Work out the finished part from the listing and answer in its coordinate system (mm). A direction names the side the tool comes from. Give positions to 0.01 mm unless a question says otherwise; leave off trailing zeros. Order: outer loops, then holes, each group sorted by start corner. A loop starts at its lowest first (then second) coordinate and runs counter-clockwise, first axis right, second up. Notation, with made-up numbers: M 80,54 L 89,54 A22 ccw 89,79 Z; hole C 30,41.5 d8. An arc over 180 degrees is marked long. One line per item, written item: value.
from build123d import *

# Parameters (mm, degrees)
EXTRUDE1_DEPTH = 9.525
SHELL1_T       = -3.175
SKETCH4_R      = 3.2729084122023364
EXTRUDE2_DEPTH = 3.175
FILLET1_R      = 6.35
FILLET2_R      = 1.016
EXTRUDE3_REACH = 99.642
SKETCH5_R      = 3.633554116992031
SKETCH5_R_2    = 2.5400000000000023
SKETCH6_R      = 2.7088319516261428
SKETCH6_R_2    = 1.739899999999999
EXTRUDE4_DEPTH = 98.64160513278141
FILLET3_R      = 0.508


with BuildPart() as part:
    # Sketch1 → Extrude1 (new body)
    with BuildSketch(Plane(origin=(0, 0, 0), x_dir=(1, 0, 0), z_dir=(0, 1, 0))):
        with BuildLine():
            Line((13.334999999999999, 0), (63.5, 0))
            Line((63.5, 0), (63.5, 38.988999999999926))
            ThreePointArc((63.5, 38.988999999999926), (60.71019209080187, 45.724192090801864), (53.97499999999993, 48.513999999999996))
            Line((53.97499999999993, 48.513999999999996), (0, 48.513999999999996))
            Line((0, 48.513999999999996), (0, 13.334999999999999))
            ThreePointArc((0, 13.334999999999999), (9.429268927122612, 9.42926892712261), (13.334999999999999, 0))
        make_face()
        with BuildLine():
            Line((25.717261934170715, 14.596576467420496), (42.82641557504918, 26.576534819151746))
            ThreePointArc((42.82641557504918, 26.576534819151746), (48.13271108628772, 25.640891752908175), (47.19706802004417, 20.334596241669633))
            Line((47.19706802004417, 20.334596241669633), (30.087914379165696, 8.354637889938386))
            ThreePointArc((30.087914379165696, 8.354637889938386), (24.78161886792715, 9.29028095618195), (25.717261934170715, 14.596576467420496))
        make_face(mode=Mode.SUBTRACT)
    extrude(amount=EXTRUDE1_DEPTH)

    # Shell1
    shell1_openings = [part.faces().sort_by_distance(p)[0] for p in [
        (38.4175, 4.7625, 0),
        (9.429268927, 4.7625, -9.429268927),
        (0, 4.7625, -30.9245),
        (32.524178478, 9.525, -25.566315858),
        (24.781618868, 4.7625, -9.290280956),
        (38.6424912, 4.7625, -14.344617066),
        (48.132711086, 4.7625, -25.640891753),
        (34.271838755, 4.7625, -20.586555643),
    ]]
    offset(amount=SHELL1_T, openings=shell1_openings, kind=Kind.INTERSECTION)

    # Sketch4 → Extrude2 (add)
    with BuildSketch(Plane(origin=(0, 0, 0), x_dir=(1, 0, 0), z_dir=(0, 1, 0))):
        with BuildLine():
            Line((41.325799999999994, 48.513999999999996), (66.82999351166346, 57.21904298473958))
            ThreePointArc((66.82999351166346, 57.21904298473958), (76.90463826764335, 54.01609142946003), (76.79370933191484, 43.445137811366784))
            Line((76.79370933191484, 43.445137811366784), (63.5, 25.8572))
            Line((63.5, 25.8572), (63.5, 38.988999999999926))
            ThreePointArc((63.5, 38.988999999999926), (60.71019209080187, 45.724192090801864), (53.97499999999993, 48.513999999999996))
            Line((53.97499999999993, 48.513999999999996), (41.325799999999994, 48.513999999999996))
        make_face()
        with Locations(Location((69.70164744855023, 48.8056189691106, 0), (0, 0, 270))):
            Circle(SKETCH4_R, mode=Mode.SUBTRACT)
    extrude(amount=EXTRUDE2_DEPTH)

    # Fillet1
    fillet1_edges = [part.edges().sort_by_distance(p)[0] for p in [
        (41.325799999999994, 1.5875, -48.513999999999996),
        (63.5, 1.5875, -25.8572),
    ]]
    fillet(fillet1_edges, radius=FILLET1_R)

    # Fillet2
    fillet2_edges = [part.edges().sort_by_distance(p)[0] for p in [
        (47.12348109415911, 3.175, -48.513999999999996),
        (26.987500000000004, 3.175, -45.339),
        (58.46512806053458, 3.175, -43.47912806053458),
        (60.325, 3.175, -19.494500000000002),
        (60.71019209080187, 3.175, -45.724192090801864),
        (63.5, 3.175, -31.358185610352162),
    ]]
    fillet(fillet2_edges, radius=FILLET2_R)

    # Sketch5 → Extrude3 (add, up to next)
    with BuildSketch(Plane(origin=(0, 4.191000000000001, 0), x_dir=(-1, 0, 0), z_dir=(0, 1, 0)), mode=Mode.PRIVATE) as extrude3_sk1:
        with Locations(Location((-53.334326567522815, -29.283102123737322, 0), (0, 0, 90))):
            Circle(SKETCH5_R)
    extrude3_tool1 = extrude(extrude3_sk1.sketch, amount=-EXTRUDE3_REACH, mode=Mode.PRIVATE) - part.part
    # Sketch5 → Extrude3 (add, up to next)
    with BuildSketch(Plane(origin=(0, 4.191000000000001, 0), x_dir=(-1, 0, 0), z_dir=(0, 1, 0)), mode=Mode.PRIVATE) as extrude3_sk2:
        with Locations(Location((-19.58000338669206, -5.648070585352799, 0), (0, 0, 90))):
            Circle(SKETCH5_R_2)
    extrude3_tool2 = extrude(extrude3_sk2.sketch, amount=-EXTRUDE3_REACH, mode=Mode.PRIVATE) - part.part
    add(extrude3_tool1.solids().sort_by_distance((53.334327, 4.191, -29.283102))[0])
    add(extrude3_tool2.solids().sort_by_distance((19.580003, 4.191, -5.648071))[0])

    # Sketch6 → Extrude4 (cut, through all)
    with BuildSketch(Plane(origin=(0, 4.191000000000001, 0), x_dir=(-1, 0, 0), z_dir=(0, 1, 0))):
        with Locations(Location((-53.334326567522815, -29.283102123737322, 0), (0, 0, 90))):
            Circle(SKETCH6_R)
        with Locations(Location((-19.58000338669206, -5.648070585352799, 0), (0, 0, 90))):
            Circle(SKETCH6_R_2)
    extrude(amount=-EXTRUDE4_DEPTH, mode=Mode.SUBTRACT)

    # Fillet3
    fillet3_edges = [part.edges().sort_by_distance(p)[0] for p in [
        (19.58000338669206, 3.175, -8.1880705853528),
        (53.334326567522815, 3.175, -32.91665624072935),
    ]]
    fillet(fillet3_edges, radius=FILLET3_R)


solid = part.part
(1) Find the intervals of material crossed by probe 1 along X at (y, z) = (3.5, -29); probe 2 along Y at (x, z) = (57, -35) (3 decimals); probe 3 along Z at (x, y) = (15, 6), in increasing order. Write a range as from..to.
Findings:
probe 1: x = 49.68..50.64, 56.03..56.99, 60.05..63.77
probe 2: y = 0..3.175
probe 3: z = -48.51..-45.34
(2) Which of the six approach directions +Z, -Z, +X, -X, +Y, -Y give full straight-line access (tool end or side, diameter ignored) to faces 1 (the cylindrical face through (49.787, 3.941, -30.071)), 2 (the flat face through (63.5, 5, -15)), 3 (the cylindrical face through (58.514, 6.821, -43.429))?
Findings:
face 1: +Y
face 2: +Z, +X, +Y
face 3: +Z, -X, +Y
(3) Section C-C, the plane y = 1 is taken. Give the vertices of the cut face in (x, z) (3 decimals), then the cut area to 3 significant figures.
Findings:
outline: M 0,-48.514 L 40.272,-48.514 A6.35 cw 42.323,-48.854 L 66.83,-57.219 A8.89 ccw 76.794,-43.445 L 64.784,-27.556 A6.35 cw 63.5,-23.727 L 63.5,0 L 13.335,0 A13.335 cw 0,-13.335 Z; hole C 19.58,-5.648 d3.48; hole M 25.717,-14.597 L 42.826,-26.577 A3.81 ccw 47.197,-20.335 L 30.088,-8.355 A3.81 ccw Z; hole C 53.334,-29.283 d5.418; hole C 69.702,-48.806 d6.546
area: 3,060 mm^2
(4) Given P1, Ø3.5, axis at x = 55, z = -27.5, coming from the +Y side; P2, Ø3, axis at y = 5, z = -51, coming from the +X side; P3, Ø4.5, axis at y = 6, z = -19, coming from the -X side; P4, Ø3, axis at y = 3.5, z = -18.5, coming from the +X side, each flat-ended and moving along its own axis, determine where each tip first touches the part or whether it passes through.
Findings:
P1: stops at y = 4.19
P2: passes through
P3: stops at x = 60.22
P4: stops at x = 63.5
(5) Section B-B, the plane x = 34 is taken. Give the vertices of the cut face in (y, z) (3 decimals), then the cut area to 3 significant figures.
Findings:
outline: M 0,-48.514 L 9.525,-48.514 L 9.525,-45.339 L 4.191,-45.339 A1.016 cw 3.175,-44.323 L 3.175,-20.396 L 0,-20.396 Z; M 0,-11.094 L 3.175,-11.094 L 3.175,0 L 0,0 Z
area: 145 mm^2
(6) Determine the mould class of faces 4 (the flat face through (27, 7, -45.339)), 5 (the cylindrical face through (17.1, 3.9, -6.2)), 6 (the flat face through (70.87, 1.57, -35.61)), 7 (the flat face through (34.15, 1.57, -20.5)) for opening direction X: pulls with the +X half, pulls with the -X half, needs draft (parallel to the pull), parting line crosses it, or undercut.
Findings:
face 4: needs draft
face 5: undercut
face 6: pulls with the +X half
face 7: undercut
(7) Section D-D, the plane x = 9 is taken. Give the vertices of the cut face in (y, z) (3 decimals).
Findings:
outline: M 0,-48.514 L 9.525,-48.514 L 9.525,-45.339 L 4.191,-45.339 A1.016 cw 3.175,-44.323 L 3.175,-9.84 L 0,-9.84 Z
(8) Section A-A, the plane y = 8.5 is taken. Give the vertices of the cut face in (x, z) (3 decimals).
Findings:
outline: M 0,-48.514 L 53.975,-48.514 A9.525 ccw 63.5,-38.989 L 63.5,0 L 60.325,0 L 60.325,-38.989 A6.35 cw 53.975,-45.339 L 0,-45.339 Z
